Work out the finished part from the listing and answer in its coordinate system (mm). Face numbers are marked on the shaded views. A direction names the side the tool comes from. Coordinates: 2 decimals unless noted, no trailing zeros. Order: outer loops, then holes, each group sorted by start corner. A loop starts at its lowest first (then second) coordinate and runs counter-clockwise, first axis right, second up. Notation, with made-up numbers: M -5.5,48 L 48.5,48 A21 ccw 48.5,85 Z; hole C 37.25,29.5 d4. An arc over 180 degrees is marked long. Use a Markdown table: item, result.
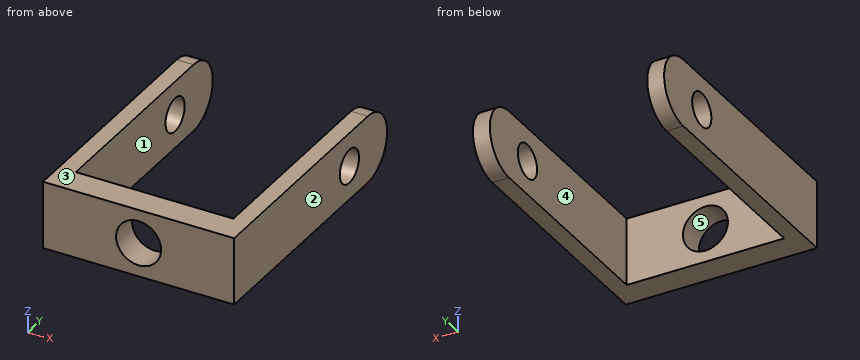
from build123d import *

# Parameters (mm, degrees)
SKETCH1_W           = 34
SKETCH1_H           = 12
BOSS_EXTRUDE1_DEPTH = 5
SKETCH5_R           = 3
BOSS_EXTRUDE3_DEPTH = 3
SKETCH6_R           = 1.5
CUT_EXTRUDE1_DEPTH  = 3
SKETCH8_R           = 4
CUT_EXTRUDE4_DEPTH  = 47.397777415


with BuildPart() as part:
    # Sketch1 → Boss-Extrude1 (new body)
    with BuildSketch(Plane(origin=(0, 0, 0), x_dir=(1, 0, 0), z_dir=(0, 1, 0))):
        Rectangle(SKETCH1_W, SKETCH1_H)
    extrude(amount=BOSS_EXTRUDE1_DEPTH)

    # Sketch5 → Boss-Extrude3 (add)
    with BuildSketch(Plane(origin=(17, 0, 0), x_dir=(0, 0, -1), z_dir=(1, 0, 0))):
        with BuildLine():
            Line((-6, 5), (6, 5))
            Line((6, 5), (6, 36))
            Line((6, 36), (6, 41.752236772))
            ThreePointArc((6, 41.752236772), (0, 47.752236772), (-6, 41.752236772))
            Line((-6, 41.752236772), (-6, 36))
            Line((-6, 36), (-6, 5))
        make_face()
        with Locations((0, 36)):
            Circle(SKETCH5_R, mode=Mode.SUBTRACT)
    boss_extrude3 = extrude(amount=-BOSS_EXTRUDE3_DEPTH)

    # Sketch6 → Cut-Extrude1 (cut)
    with BuildSketch(Plane(origin=(0, 5, 0), x_dir=(1, 0, 0), z_dir=(0, 1, 0))):
        with Locations(Location((0, 0, 0), (0, 0, 270))):
            Circle(SKETCH6_R)
    extrude(amount=-CUT_EXTRUDE1_DEPTH, mode=Mode.SUBTRACT)

    # Sketch8 → Cut-Extrude4 (cut, through all)
    with BuildSketch(Plane(origin=(0, 5, 0), x_dir=(1, 0, 0), z_dir=(0, 1, 0))):
        with Locations(Location((0, 0, 0), (0, 0, 270))):
            Circle(SKETCH8_R)
    extrude(amount=-CUT_EXTRUDE4_DEPTH, mode=Mode.SUBTRACT)

    # Mirror1: Boss-Extrude3 across plane
    add(boss_extrude3.mirror(Plane(origin=(0, 0, 0), x_dir=(0, 0, 1), z_dir=(1, 0, 0))))


solid = part.part
(1) Given P1, Ø2, axis at x = 0, z = -2.5, coming from the -Y side; P2, Ø5, axis at x = -1, z = 4, coming from the +Y side, each flat-ended and moving along its own axis, determine where each tip first touches the part or whether it passes through.
Conclusion:
| item | result |
|---|---|
| P1 | through |
| P2 | y = 5 |
(2) Straight lines are drawn through the part: L1, parallel to X at y = 31, z = 0.5; L2, parallel to X at y = 2.85, z = 0; L3, parallel to Y at x = -15.95, z = 0. For each, find the intervals that lie inside material, in ascending order.
Conclusion:
| item | result |
|---|---|
| L1 | -17 to -14, 14 to 17 |
| L2 | -17 to -4, 4 to 17 |
| L3 | 0 to 33, 39 to 47.75 |
(3) A cutting plane is placed at D-D (y = 29.5). Determine the outline of the cut face in (x, z).
Conclusion:
| item | result |
|---|---|
| outline | M -17,-6 L -14,-6 L -14,6 L -17,6 Z; M 14,-6 L 17,-6 L 17,6 L 14,6 Z |
(4) A cutting plane is placed at A-A (y = 36). Determine the outline of the cut face in (x, z).
Conclusion:
| item | result |
|---|---|
| outline | M -17,-6 L -14,-6 L -14,-3 L -17,-3 Z; M -17,3 L -14,3 L -14,6 L -17,6 Z; M 14,-6 L 17,-6 L 17,-3 L 14,-3 Z; M 14,3 L 17,3 L 17,6 L 14,6 Z |
(5) Which of the six approach directions +Z, -Z, +X, -X, +Y, -Y give full straight-line access (tool end or side, diameter ignored) to the marked faces 4 and 5?
Conclusion:
| item | result |
|---|---|
| face 4 | +Z, -Z, +Y |
| face 5 | +Y, -Y |
(6) A cutting plane is placed at C-C (z = 0). Determine the outline of the cut face in (x, y), then the cut area to 3 significant figures.
Conclusion:
| item | result |
|---|---|
| outline | M -17,0 L -4,0 L -4,5 L -14,5 L -14,33 L -17,33 Z; M -17,39 L -14,39 L -14,47.75 L -17,47.75 Z; M 4,0 L 17,0 L 17,33 L 14,33 L 14,5 L 4,5 Z; M 14,39 L 17,39 L 17,47.75 L 14,47.75 Z |
| area | 351 mm2 |
(7) Determine the mould class of the marked faces 1, 2 and 3 for opening direction X: pulls with the +X half, pulls with the -X half, needs draft (parallel to the pull), parting line crosses it, or undercut.
Conclusion:
| item | result |
|---|---|
| face 1 | undercut |
| face 2 | pulls with the +X half |
| face 3 | needs draft |
(8) A cutting plane is placed at B-B (x = 0). Determine the outline of the cut face in (y, z).
Conclusion:
| item | result |
|---|---|
| outline | M 0,-6 L 5,-6 L 5,-4 L 0,-4 Z; M 0,4 L 5,4 L 5,6 L 0,6 Z |
